The listing builds one solid part. Answer for the finished solid, in the listing's coordinates (mm). Face numbers are marked on the shaded views. A direction names the side the tool comes from. Coordinates: 2 decimals unless noted, no trailing zeros. Write each loop counter-clockwise with the first axis right and the second up, starting at its lowest first coordinate (ties: lowest second). Pieces come first, ordered by that corner, then holes.
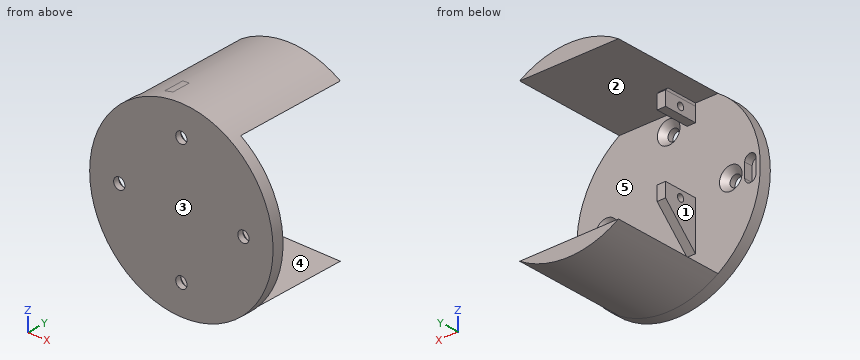
from build123d import *
from build123d.topology import SkipClean

# Parameters (mm, degrees)
SKETCH1_R           = 32.5
SKETCH1_R_2         = 2
BOSS_EXTRUDE1_DEPTH = 4
BOSS_EXTRUDE2_DEPTH = 40
CHAMFER1_SIZE       = 2
SKETCH3_W           = 3
SKETCH3_H           = 5
BOSS_EXTRUDE3_DEPTH = 12
SKETCH4_R           = 1.25
CUT_EXTRUDE1_DEPTH  = 3
CUT_EXTRUDE2_DEPTH  = 3
CHAMFER3_SIZE       = 12


with BuildPart() as part:
    # Sketch1 → Boss-Extrude1 (new body)
    with BuildSketch(Plane(origin=(0, 0, 0), x_dir=(1, 0, 0), z_dir=(0, 1, 0))):
        with Locations(Location((0, 0, 0), (0, 0, 270))):
            Circle(SKETCH1_R)
        with Locations(Location((-22, 0, 0), (0, 0, 270))):
            Circle(SKETCH1_R_2, mode=Mode.SUBTRACT)
        with Locations(Location((0, 22, 0), (0, 0, 270))):
            Circle(SKETCH1_R_2, mode=Mode.SUBTRACT)
        with Locations(Location((22, 0, 0), (0, 0, 270))):
            Circle(SKETCH1_R_2, mode=Mode.SUBTRACT)
        with Locations(Location((0, -22, 0), (0, 0, 270))):
            Circle(SKETCH1_R_2, mode=Mode.SUBTRACT)
    extrude(amount=BOSS_EXTRUDE1_DEPTH)

    # Sketch2 → Boss-Extrude2 (add)
    with SkipClean():  # the faces are left unmerged after this step: merging them gives an invalid solid
        with BuildSketch(Plane(origin=(0, 4, 0), x_dir=(1, 0, 0), z_dir=(0, 1, 0))):
            with BuildLine():
                Line((17.5, 27.386127875), (-17.5, 27.386127875))
                ThreePointArc((-17.5, 27.386127875), (0, 32.5), (17.5, 27.386127875))
            make_face()
            with BuildLine():
                Line((17.5, -27.386127875), (-17.5, -27.386127875))
                ThreePointArc((-17.5, -27.386127875), (0, -32.5), (17.5, -27.386127875))
            make_face()
        extrude(amount=BOSS_EXTRUDE2_DEPTH)

    # Chamfer1
    chamfer1_edges = [part.edges().sort_by_distance(p)[0] for p in [
        (22, 4, -2),
        (0, 4, 20),
        (-22, 4, -2),
        (0, 4, -24),
    ]]
    chamfer(chamfer1_edges, length=CHAMFER1_SIZE)

    # Sketch3 → Boss-Extrude3 (add)
    with SkipClean():  # the faces are left unmerged after this step: merging them gives an invalid solid
        with BuildSketch(Plane(origin=(0, 4, 0), x_dir=(1, 0, 0), z_dir=(0, 1, 0))):
            with Locations((-8, 3.9)):
                Rectangle(SKETCH3_W, SKETCH3_H)
            with Locations((-8, -23.9)):
                Rectangle(SKETCH3_W, SKETCH3_H)
        extrude(amount=BOSS_EXTRUDE3_DEPTH)

    # Sketch4 → Cut-Extrude1 (cut)
    with SkipClean():  # the faces are left unmerged after this step: merging them gives an invalid solid
        with BuildSketch(Plane.ZY.offset(9.5)):
            with Locations((-3.9, 10)):
                Circle(SKETCH4_R)
            with Locations((23.9, 10)):
                Circle(SKETCH4_R)
        extrude(amount=-CUT_EXTRUDE1_DEPTH, mode=Mode.SUBTRACT)

    # Sketch5 → Cut-Extrude2 (cut)
    with SkipClean():  # the faces are left unmerged after this step: merging them gives an invalid solid
        with BuildSketch(Plane(origin=(0, 4, 0), x_dir=(1, 0, 0), z_dir=(0, 1, 0))):
            with BuildLine():
                Line((-30.95, 1.9), (-30.95, -3.1))
                ThreePointArc((-30.95, -3.1), (-28.95, -5.1), (-26.95, -3.1))
                Line((-26.95, -3.1), (-26.95, 1.9))
                ThreePointArc((-26.95, 1.9), (-28.95, 3.9), (-30.95, 1.9))
            make_face()
        extrude(amount=-CUT_EXTRUDE2_DEPTH, mode=Mode.SUBTRACT)

    # Chamfer3
    # the kernel refuses this chamfer: 12 mm, written as the material it adds along each edge
    with BuildSketch(Plane(origin=(-9.5, 4, -6.4), x_dir=(0, -0.02749587661058638, -0.9996219169112968), z_dir=(1, 0, 0))) as chamfer3_piece_1_section:
        Polygon((CHAMFER3_SIZE * 0.999621916911, CHAMFER3_SIZE * 0.0274958766106), (-CHAMFER3_SIZE * 0.0274958766106, CHAMFER3_SIZE * 0.999621916911), (0, 0), align=None)
    chamfer3_piece_1 = extrude(amount=3, mode=Mode.PRIVATE)
    chamfer3_piece_1 = split(chamfer3_piece_1, bisect_by=Plane(origin=(-8, 16, -10.364849852), z_dir=(0, -1, 0)), keep=Keep.TOP, mode=Mode.PRIVATE)
    add(chamfer3_piece_1)
    with BuildSketch(Plane(origin=(-6.5, 4, 26.4), x_dir=(-1.1837901526131805e-15, -0.027495876610586386, 0.9996219169112968), z_dir=(-1, 0, 0))) as chamfer3_piece_2_section:
        Polygon((CHAMFER3_SIZE * 0.999621916911, CHAMFER3_SIZE * 0.0274958766106), (-CHAMFER3_SIZE * 0.0274958766106, CHAMFER3_SIZE * 0.999621916911), (0, 0), align=None)
    chamfer3_piece_2 = extrude(amount=3, mode=Mode.PRIVATE)
    chamfer3_piece_2 = chamfer3_piece_2 & Plane(origin=(0, 8.886128488, 0), x_dir=(0, 0, 1), z_dir=(0, -1, 0)) * Cylinder(32.5, 54, mode=Mode.PRIVATE)
    chamfer3_piece_2 = split(chamfer3_piece_2, bisect_by=Plane(origin=(-7.974151993, 16, 28.556689734), z_dir=(0, -1, 0)), keep=Keep.TOP, mode=Mode.PRIVATE)
    add(chamfer3_piece_2)


solid = part.part
Q1. The part is cut by section D-D, the plane x = 14. Write down the section's boundary in (y, z), then the cut area to 3 significant figures.
Answers below:
outline: (0, -29.33) - (44, -29.33) - (44, -27.39) - (4, -27.39) - (4, 27.39) - (44, 27.39) - (44, 29.33) - (0, 29.33) - close
area: 390 mm2
Q2. Determine the mould class of the marked faces 1, 2 and 3 for opening direction Z: released by +Z, released by -Z, zero draft, split by the parting line, or undercut.
Answers below:
face 1: undercut
face 2: undercut
face 3: zero draft
Q3. The part is cut by section C-C, the plane y = 39.5. Write down the section's boundary in (x, z).
Answers below:
outline: (-17.5, -27.39) arc R32.5 ccw to (17.5, -27.39) - close; (-17.5, 27.39) - (17.5, 27.39) arc R32.5 ccw to start
Q4. The part is cut by section A-A, the plane x = 22. Write down the section's boundary in (y, z), then the cut area to 3 significant figures.
Answers below:
outline: (0, -23.92) - (4, -23.92) - (4, -4) - (2, -2) - (0, -2) - close; (0, 2) - (2, 2) - (4, 4) - (4, 23.92) - (0, 23.92) - close
area: 171 mm2
Q5. Given pin 1 (5.5 mm diameter, centred on y = 7.5, z = 24.5, fed in from +X); pin 2 (8 mm diameter, centred on y = 9.5, z = -25, fed in from +X); pin 3 (3 mm diameter, centred on y = 10, z = 23.9, fed in from -X); pin 4 (5 mm diameter, centred on x = -19.5, z = -21, fed in from -Y), each flat-ended and moving along its own axis, determine where each tip first touches the part or whether it passes through.
Answers below:
pin 1: stops at x = -6.5
pin 2: stops at x = 17.5
pin 3: stops at x = -9.5
pin 4: stops at y = 0
Q6. The part is cut by section B-B, the plane z = -22. Write down the section's boundary in (x, y), then the cut area to 3 significant figures.
Answers below:
outline: (-23.92, 0) - (-2, 0) - (-2, 2) - (-4, 4) - (-23.92, 4) - close; (2, 0) - (23.92, 0) - (23.92, 4) - (4, 4) - (2, 2) - close
area: 171 mm2
Q7. Which of the six approach directions +Z, -Z, +X, -X, +Y, -Y give full straight-line access (tool end or side, diameter ignored) to the marked faces 4 and 5?
Answers below:
face 4: +X, -X, +Y
face 5: +Y
Q8. Find the intervals of material crossed by probe 1 along X at (y, z) = (1.2, 0); probe 2 along X at (y, z) = (0.95, 0); probe 3 along Y at (x, z) = (13, -18), in increasing order.
Answers below:
probe 1: x = -32.5 to -30.95, -26.95 to -24, -20 to 20, 24 to 32.5
probe 2: x = -32.5 to -24, -20 to 20, 24 to 32.5
probe 3: y = 0 to 4
